Study the drawing (mm; zero at the part's minimum x, y, z) and answer. Round coordinates to 2 decimals unless told otherwise and drop trailing zeros. Write each loop counter-clockwise with the first axis right and the second up, starting at its lowest first coordinate (ties: lowest second). Pieces come first, ordered by that corner, then holes.
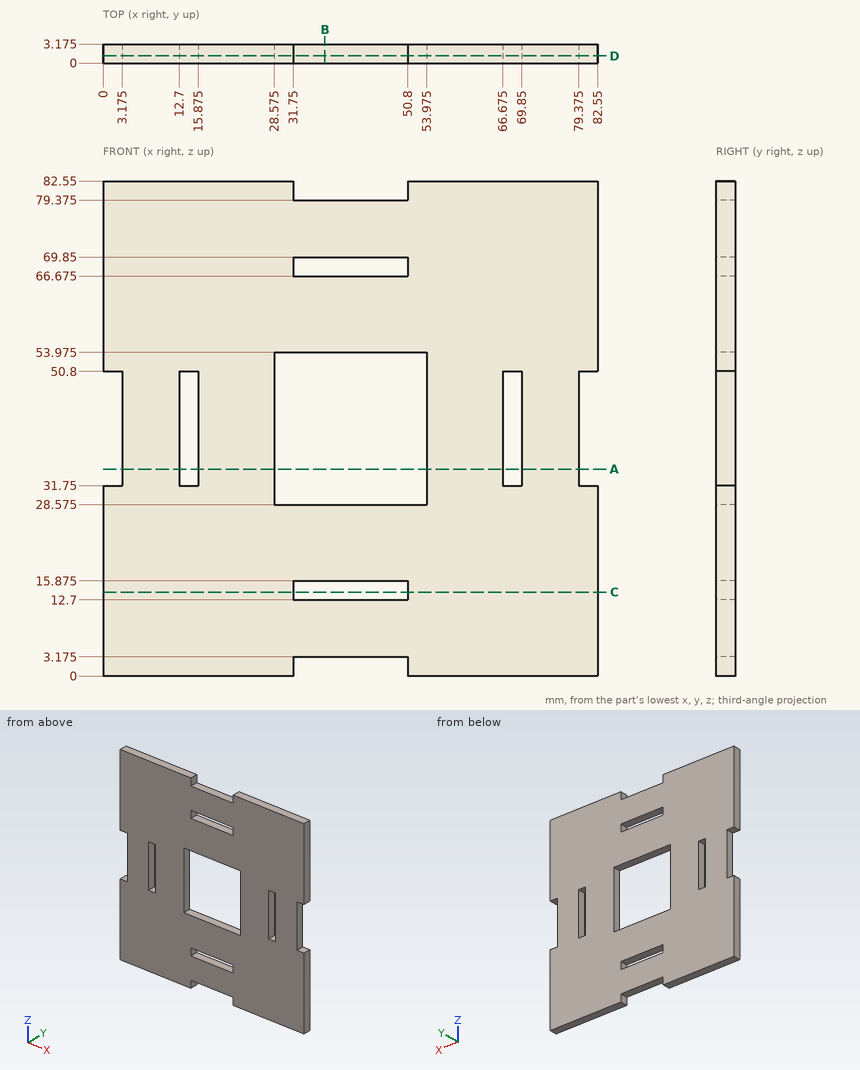
1. Section C-C on z = 14 is taken. Determine the outline of the cut face in (x, y) (3 decimals), plus the area to 3 significant figures.
Geometry says:
outline: (0, 0) - (31.75, 0) - (31.75, 3.175) - (0, 3.175) - close; (50.8, 0) - (82.55, 0) - (82.55, 3.175) - (50.8, 3.175) - close
area: 202 mm2
2. Section B-B on x = 37 is taken. Determine the outline of the cut face in (y, z) (3 decimals), plus the area to 3 significant figures.
Geometry says:
outline: (0, 3.175) - (3.175, 3.175) - (3.175, 12.7) - (0, 12.7) - close; (0, 15.875) - (3.175, 15.875) - (3.175, 28.575) - (0, 28.575) - close; (0, 53.975) - (3.175, 53.975) - (3.175, 66.675) - (0, 66.675) - close; (0, 69.85) - (3.175, 69.85) - (3.175, 79.375) - (0, 79.375) - close
area: 141 mm2
3. Section D-D on y = 1.2 is taken. Give the number of separate pieces and of enclosed holes in the cut face, plus the area to 3 significant figures.
Geometry says:
separate pieces: 1
enclosed holes: 5
area: 5,690 mm2
4. Straight lines are drawn through the part: line 1 along X through (y, z) = (0.3, 36) (3 decimals); line 2 along X through (y, z) = (2.2, 14.5). For each, find the intervals that lie inside material, in ascending order.
Geometry says:
line 1: x = 3.175 to 12.7, 15.875 to 28.575, 53.975 to 66.675, 69.85 to 79.375
line 2: x = 0 to 31.75, 50.8 to 82.55
5. Given pin 1 (1 mm diameter, centred on y = 1.5, z = 37.5, fed in from -X) (3 decimals); pin 2 (1 mm diameter, centred on x = 35.5, y = 1, fed in from +Z) (3 decimals); pin 3 (12 mm diameter, centred on x = 35, z = 39, fed in from +Y); pin 4 (1 mm diameter, centred on y = 2, z = 37, fed in from +X) (3 decimals), each flat-ended and moving along its own axis, determine where each tip first touches the part or whether it passes through.
Geometry says:
pin 1: stops at x = 3.175
pin 2: stops at z = 79.375
pin 3: passes through
pin 4: stops at x = 79.375
6. Section A-A on z = 34.5 is taken. Determine the outline of the cut face in (x, y) (3 decimals), plus the area to 3 significant figures.
Geometry says:
outline: (3.175, 0) - (12.7, 0) - (12.7, 3.175) - (3.175, 3.175) - close; (15.875, 0) - (28.575, 0) - (28.575, 3.175) - (15.875, 3.175) - close; (53.975, 0) - (66.675, 0) - (66.675, 3.175) - (53.975, 3.175) - close; (69.85, 0) - (79.375, 0) - (79.375, 3.175) - (69.85, 3.175) - close
area: 141 mm2
